Geometry check sheet. Reference: the model listing, model coordinates, mm. Face numbers are marked on the shaded views. A direction names the side the tool comes from. Coordinates: 2 decimals unless noted, no trailing zeros. Order: outer loops, then holes, each group sorted by start corner. A loop starts at its lowest first (then second) coordinate and runs counter-clockwise, first axis right, second up. Notation, with made-up numbers: (-2, -19) - (14, -19) arc R6 cw to (14, -12) - close; hole circle Ø3 at (-6, 44.5). An arc over 180 degrees is marked (long way). Return JSON: item names as keys, results as strings. Group by question number.
Item 1: Section check C-C on x = 32. Enter the section's corners in (y, z).
Item 2: Scan lines: probe 1 along X at (y, z) = (1.35, -21.5); probe 2 along Z at (x, y) = (38, 0.25); probe 3 along Z at (x, y) = (26, -2.75). Record each from-to range of solid material in increasing order.
Item 3: Section check A-A on y = 4.5. Enter the section's corners in (x, z), then the cut area to 3 significant figures.
Item 4: Tool access check on the marked faces 1, 2 and 3. Record the directions out of +Z, -Z, +X, -X, +Y, -Y that give a thin tool (end or side, any length) a straight path to the whole face; none if there is none.
Item 5: Gauge pin test, flat ends, axial feed: pin 1 (1 mm diameter, centred on x = 30, y = -1, fed in from -Z); pin 2 (25 mm diameter, centred on x = -11, z = -4.5, fed in from -Y); pin 3 (5 mm diameter, centred on x = 29.5, z = 21, fed in from +Y); pin 4 (2.5 mm diameter, centred on x = 39, z = 21.5, fed in from +Y). Record the tip position at first contact, or that the pin passes through.
Item 6: Section check D-D on y = 8.5. Enter the section's corners in (x, z), then the cut area to 3 significant figures.
Item 7: Section check B-B on z = 8.5. Enter the section's corners in (x, y), then the cut area to 3 significant figures.
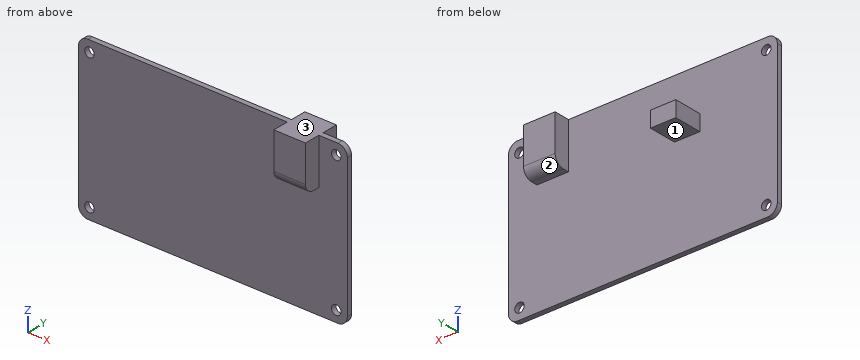
from build123d import *

# Parameters (mm, degrees)
SKETCH_1_W      = 85
SKETCH_1_H      = 50
SKETCH_1_R      = 1.5
EXTRUDE_1_DEPTH = 1.6
FILLET_1_R      = 3
SKETCH_2_W      = 10
SKETCH_2_H      = 14.5
EXTRUDE_2_DEPTH = 5
SKETCH_3_W      = 8
SKETCH_3_H      = 5
EXTRUDE_3_DEPTH = 9
SKETCH_4_W      = 10
SKETCH_4_H      = 14.5
EXTRUDE_4_DEPTH = 5
FILLET_2_R      = 3


with BuildPart() as part:
    # 草图1 → 凸台-拉伸1 (new body)
    with BuildSketch(Plane(origin=(0, 0, 0), x_dir=(1, 0, 0), z_dir=(0, 1, 0))):
        Rectangle(SKETCH_1_W, SKETCH_1_H)
        with Locations(Location((-39, 21.5, 0), (0, 0, 270))):
            Circle(SKETCH_1_R, mode=Mode.SUBTRACT)
        with Locations(Location((39, 21.5, 0), (0, 0, 270))):
            Circle(SKETCH_1_R, mode=Mode.SUBTRACT)
        with Locations(Location((39, -21.5, 0), (0, 0, 270))):
            Circle(SKETCH_1_R, mode=Mode.SUBTRACT)
        with Locations(Location((-39, -21.5, 0), (0, 0, 270))):
            Circle(SKETCH_1_R, mode=Mode.SUBTRACT)
    extrude(amount=EXTRUDE_1_DEPTH)

    # 圆角1
    fillet_1_edges = [part.edges().sort_by_distance(p)[0] for p in [
        (42.5, 0.8, 25),
        (-42.5, 0.8, 25),
        (-42.5, 0.8, -25),
        (42.5, 0.8, -25),
    ]]
    fillet(fillet_1_edges, radius=FILLET_1_R)

    # 草图2 → 凸台-拉伸2 (add)
    with BuildSketch(Plane(origin=(0, 1.6, 0), x_dir=(1, 0, 0), z_dir=(0, 1, 0))):
        with Locations((28.5, -17.75)):
            Rectangle(SKETCH_2_W, SKETCH_2_H)
    extrude(amount=EXTRUDE_2_DEPTH)

    # 草图3 → 凸台-拉伸3 (add)
    with BuildSketch(Plane(origin=(0, 1.6, 0), x_dir=(1, 0, 0), z_dir=(0, 1, 0))):
        with Locations((-14, -9)):
            Rectangle(SKETCH_3_W, SKETCH_3_H)
    extrude(amount=EXTRUDE_3_DEPTH)

    # 草图4 → 凸台-拉伸4 (add)
    with BuildSketch(Plane.XZ):
        with Locations((28.5, 17.75)):
            Rectangle(SKETCH_4_W, SKETCH_4_H)
    extrude(amount=EXTRUDE_4_DEPTH)

    # 圆角2
    fillet_2_edges = [part.edges().sort_by_distance(p)[0] for p in [
        (28.5, 6.6, 10.5),
        (28.5, -5, 10.5),
    ]]
    fillet(fillet_2_edges, radius=FILLET_2_R)


solid = part.part
Computed:
{
 "1": {"outline": "(-5, 13.5) arc R3 ccw to (-2, 10.5) - (0, 10.5) - (0, -25) - (1.6, -25) - (1.6, 10.5) - (3.6, 10.5) arc R3 ccw to (6.6, 13.5) - (6.6, 25) - (-5, 25) - close"},
 "2": {"probe 1": "x = -42.5 to -40.5, -37.5 to 37.5, 40.5 to 42.5", "probe 2": "z = -25 to -22.62, -20.38 to 20.38, 22.62 to 25", "probe 3": "z = 10.6 to 25"},
 "3": {"outline": "(-18, 6.5) - (-10, 6.5) - (-10, 11.5) - (-18, 11.5) - close; (23.5, 10.64) - (33.5, 10.64) - (33.5, 25) - (23.5, 25) - close", "area": "184 mm²"},
 "4": {"face 1": "-Z, +X, -X, +Y", "face 2": "-Z, +X, +Y", "face 3": "+Z, +X, -X, +Y, -Y"},
 "5": {"pin 1": "stops at z = 10.5", "pin 2": "stops at y = 0", "pin 3": "stops at y = 6.6", "pin 4": "passes through"},
 "6": {"outline": "(-18, 6.5) - (-10, 6.5) - (-10, 11.5) - (-18, 11.5) - close", "area": "40.0 mm²"},
 "7": {"outline": "(-42.5, 0) - (42.5, 0) - (42.5, 1.6) - (-10, 1.6) - (-10, 10.6) - (-18, 10.6) - (-18, 1.6) - (-42.5, 1.6) - close", "area": "208 mm²"}
}
